```python
from build123d import *

# Parameters (mm, degrees)
F0_W     = 40
F0_H     = 36
F1_DEPTH = 12
F2_T     = -2
F3_R     = 6
F4_DEPTH = 25
F5_R     = 1


with BuildPart() as f1:
    # F0 (on Front) → F1 (new body)
    with BuildSketch(Plane.XZ):
        with Locations((20, 18)):
            Rectangle(F0_W, F0_H)
    extrude(amount=F1_DEPTH)

    # F2
    f2_openings = [f1.faces().sort_by_distance(p)[0] for p in [
        (20, -12, 18),
    ]]
    offset(amount=F2_T, openings=f2_openings)

    # F3 (on face) → F4 (cut)
    with BuildSketch(Plane(origin=(0, 0, 0), x_dir=(-1, 0, 0), z_dir=(0, 1, 0))):
        with Locations((-20, 18)):
            Circle(F3_R)
    extrude(amount=-F4_DEPTH, mode=Mode.SUBTRACT)

    # F5
    f5_edges = [f1.edges().sort_by_distance(p)[0] for p in [
        (40, -6, 0),
        (40, -6, 36),
        (0, -6, 0),
        (0, -6, 36),
    ]]
    fillet(f5_edges, radius=F5_R)


solid = f1.part
```
Build history of the part. All positions in model axes, mm. A direction names the side the tool comes from. Give positions to 0.01 mm unless a question says otherwise; leave off trailing zeros. Loops run counter-clockwise (first coordinate to the right, second up) from the corner with the lowest first, then second, coordinate; pieces in that order, holes last. Notation, with made-up numbers: (18.5, 34.25) - (60.5, 34.25) arc R9 cw to (60.5, 42.25) - close; hole circle Ø10 at (33, 56). An arc over 180 degrees is marked (long way). Use a Markdown table: item, result.
(1) Pull direction Z, two halves, no side cores. Call faces 3 (the face through (0, -6, 18)), 4 (the face through (24.76, -0.99, 14.35)), 5 (the face through (20, -7, 2)), 6 (the face through (0.285, -6.084, 0.301)): +Z half, -Z half, draft (parallel to the pull), parting line (faces both ways), or undercut.
Taken from the geometry:
| item | result |
|---|---|
| face 3 | draft |
| face 4 | undercut |
| face 5 | undercut |
| face 6 | -Z half |
(2) Drop flat-ended pins along their axis: pin 1 Ø2 at (x, z) = (25.5, 10) entering from +Y; pin 2 Ø15.5 at (x, z) = (20, 18) entering from -Y. Give the stop position or say it passes through.
Taken from the geometry:
| item | result |
|---|---|
| pin 1 | y = 0 |
| pin 2 | y = -2 |
(3) Band-saw the part on D-D (x = 7). Give the cut face in (y, z), and give its area (3 significant figures).
Taken from the geometry:
| item | result |
|---|---|
| outline | (-12, 0) - (0, 0) - (0, 36) - (-12, 36) - (-12, 34) - (-2, 34) - (-2, 2) - (-12, 2) - close |
| area | 112 mm2 |
(4) Band-saw the part on B-B (x = 20). Give the cut face in (y, z), and give its area (3 significant figures).
Taken from the geometry:
| item | result |
|---|---|
| outline | (-12, 0) - (0, 0) - (0, 12) - (-2, 12) - (-2, 2) - (-12, 2) - close; (-12, 34) - (-2, 34) - (-2, 24) - (0, 24) - (0, 36) - (-12, 36) - close |
| area | 88.0 mm2 |
(5) Band-saw the part on C-C (y = -1.5). Give the cut face in (x, z).
Taken from the geometry:
| item | result |
|---|---|
| outline | (0, 1) arc R1 ccw to (1, 0) - (39, 0) arc R1 ccw to (40, 1) - (40, 35) arc R1 ccw to (39, 36) - (1, 36) arc R1 ccw to (0, 35) - close; hole circle Ø12 at (20, 18) |
(6) Band-saw the part on A-A (z = 18). Give the cut face in (x, y), and give its area (3 significant figures).
Taken from the geometry:
| item | result |
|---|---|
| outline | (0, -12) - (2, -12) - (2, -2) - (14, -2) - (14, 0) - (0, 0) - close; (26, -2) - (38, -2) - (38, -12) - (40, -12) - (40, 0) - (26, 0) - close |
| area | 96.0 mm2 |
(7) Wall check: line 1 along Z through (x, y) = (22.5, -9.5); line 2 along X through (y, z) = (-2.5, 3.5); line 3 along Z through (x, y) = (20, -1.6). Give the ranges that are in metal, low to high.
Taken from the geometry:
| item | result |
|---|---|
| line 1 | 0 to 2, 34 to 36 |
| line 2 | 0 to 2, 38 to 40 |
| line 3 | 0 to 12, 24 to 36 |
(8) Which spindle directions (+Z, -Z, +X, -X, +Y, -Y) get a long thin tool onto all of the face, cutting with end or side? Do faces 1 (the face through (40, -6, 18)), 2 (the face through (20, -7, 34)). Say none if no direction does.
Taken from the geometry:
| item | result |
|---|---|
| face 1 | +Z, -Z, +X, +Y, -Y |
| face 2 | -Y |
